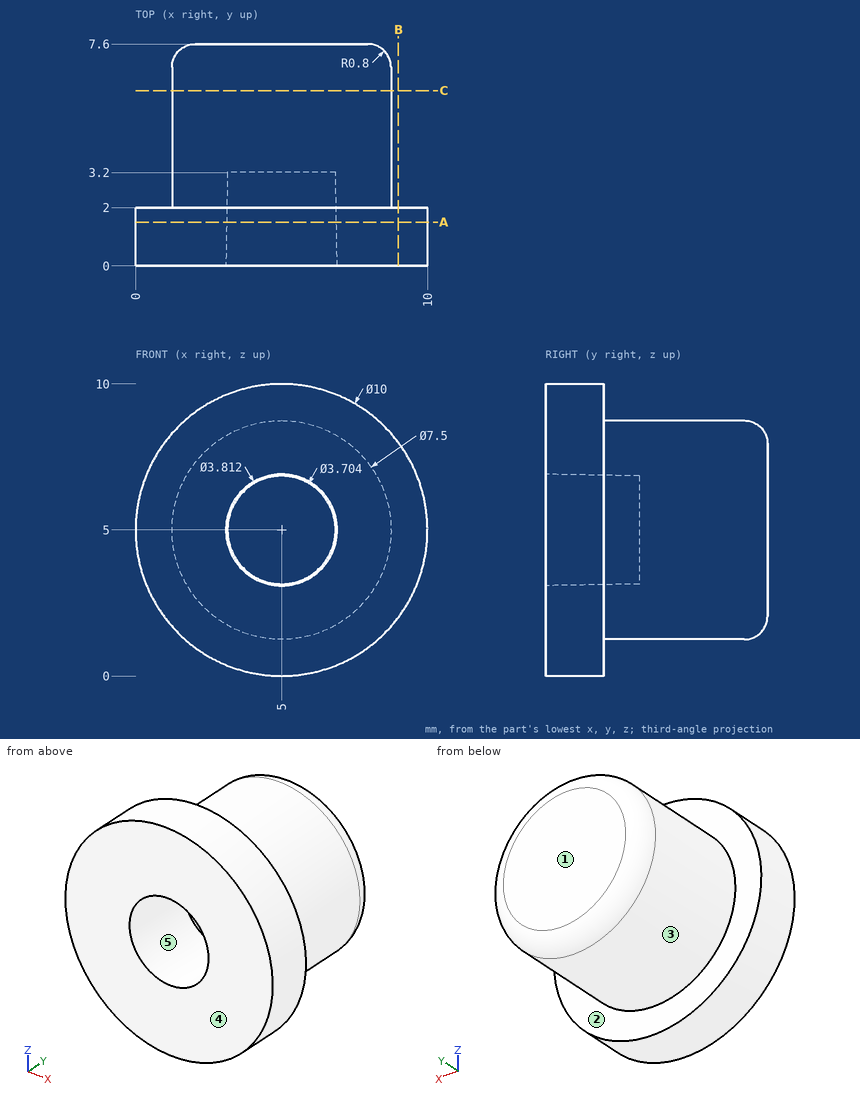
Study the drawing (mm; zero at the part's minimum x, y, z) and answer. A direction names the side the tool comes from. Coordinates: 2 decimals unless noted, no trailing zeros. Loops run counter-clockwise (first coordinate to the right, second up) from the corner with the lowest first, then second, coordinate; pieces in that order, holes last. Notation, with made-up numbers: M 57,19.25 L 115,19.25 A12 ccw 115,23.25 Z; hole C 35,-20.5 d8. An arc over 180 degrees is marked long. Answer as a JSON object with one key per item and string values. Group by question number.
Item 1: Each of these flat-tipped pins is pushed along its axis until it touches: P1, Ø2, axis at x = 1.5, z = 8.5, coming from the +Y side; P2, Ø4, axis at x = 5.5, y = 2, coming from the +Z side; P3, Ø1, axis at x = 4, y = 4, coming from the +Z side; P4, Ø1.5, axis at y = 2.5, z = 6, coming from the +X side. Where does it stop, or does it pass through?
Item 2: Section C-C (y = 6) is taken. Write down the section's boundary in (x, z).
Item 3: Which of the six approach directions +Z, -Z, +X, -X, +Y, -Y give full straight-line access (tool end or side, diameter ignored) to the marked faces 1 and 2?
Item 4: Section B-B (x = 9) is taken. Write down the section's boundary in (y, z), and give its area (3 significant figures).
Item 5: Determine the mould class of the marked faces 3, 4 and 5 for opening direction X: +X half, -X half, draft (parallel to the pull), parting line (faces both ways), or undercut.
Item 6: Section A-A (y = 1.5) is taken. Write down the section's boundary in (x, z).
Item 7: Consider L1, parallel to Y at x = 1.5, z = 7.5; L2, parallel to Y at x = 4, z = 5.5; L3, parallel to Z at x = 3.5, y = 1.5 (1 decimal). Determine where each line is inside the solid, lowest interval first.
Solved:
{
 "1": {"P1": "stops at y = 2", "P2": "stops at z = 10", "P3": "stops at z = 8.72", "P4": "stops at x = 9.98"},
 "2": {"outline": "C 5,5 d7.5"},
 "3": {"face 1": "+Z, -Z, +X, -X, +Y", "face 2": "+Y"},
 "4": {"outline": "M 0,2 L 2,2 L 2,8 L 0,8 Z", "area": "12.0 mm2"},
 "5": {"face 3": "parting line", "face 4": "draft", "face 5": "undercut"},
 "6": {"outline": "C 5,5 d10; hole C 5,5 d3.76"},
 "7": {"L1": "y = 0 to 2", "L2": "y = 3.2 to 7.6", "L3": "z = 0.2 to 3.9, 6.1 to 9.8"}
}
